```python
from build123d import *

# Parameters (mm, degrees)
F0_R     = 25.4
F1_DEPTH = 5.08
F3_DEPTH = 12.7
F4_R     = 1.5875
F5_DEPTH = 25.4


with BuildPart() as f1:
    # F0 (on Top) → F1 (new body)
    with BuildSketch(Plane.XY):
        Circle(F0_R)
    extrude(amount=F1_DEPTH)

    # F2 (on face) → F3 (join)
    with BuildSketch(Plane.XY.offset(5.08)):
        with BuildLine():
            ThreePointArc((13.335, 0), (0, -13.335), (-13.335, 0))
            Line((-13.335, 0), (-13.335, 12.7))
            ThreePointArc((-13.335, 12.7), (0, -18.415), (13.335, 12.7))
            Line((13.335, 12.7), (13.335, 0))
        make_face()
    extrude(amount=F3_DEPTH)

    # F4 (on face) → F5 (cut)
    with BuildSketch(Plane.XY.offset(5.08)):
        with Locations((-21.9075, 0)):
            Circle(F4_R)
        with Locations((21.9075, 0)):
            Circle(F4_R)
        with Locations((0, -21.9075)):
            Circle(F4_R)
    extrude(amount=-F5_DEPTH, mode=Mode.SUBTRACT)


solid = f1.part
```
Here's how the part is built. I have some questions about the finished solid (model axes, mm). A direction names the side the tool comes from. Round coordinates to 2 decimals unless told otherwise and drop trailing zeros. Loops run counter-clockwise (first coordinate to the right, second up) from the corner with the lowest first, then second, coordinate; pieces in that order, holes last. Notation, with made-up numbers: (44, 32) -> (69, 32) arc R21 ccw to (69, 52) -> close; hole circle Ø9 at (55.5, 27). An arc over 180 degrees is marked (long way). Answer as CSV lines item,"result". Start each with the question number.
1. Imagine slicing it at A-A on x = 0. Write out the boundary of the cut face in (y, z) (3 decimals), plus the area to 3 significant figures.
2. For faces 1 (the face through (13.335, 6, 11)), 2 (the face through (23.42, 0.48, 2.58)), 3 (the face through (-0.601, -18.405, 11.341)), which set-ups out of +Z, -Z, +X, -X, +Y, -Y let a thin tool reach every point of the face, with its end or its side?
3. Imagine slicing it at C-C on z = 11.5. Write out the boundary of the cut face in (x, y) (3 decimals), plus the area to 3 significant figures.
4. Imagine slicing it at B-B on y = 12. Write out the boundary of the cut face in (x, z) (3 decimals).
5. I need wall thicknesses on probe 1 along X at (y, z) = (-1, 2); probe 2 along Y at (x, z) = (0, 3.35) (3 decimals); probe 3 along Z at (x, y) = (5.5, 9.5). Which ranges of each line are inside material? Lowest first, please. Write a range as from..to.
6. I'm going to push flat-ended pins straight in: P1, Ø4, axis at y = 4, z = 7, coming from the -X side; P2, Ø2.5, axis at x = 0, y = -21.91, coming from the -Z side; P3, Ø8, axis at y = -9.5, z = 13, coming from the -X side; P4, Ø10, axis at x = -8.5, z = 3.5, coming from the +Y side. Where does each tip first touch, or does it pass through?
7. Imagine slicing it at D-D on x = -22. Write out the boundary of the cut face in (y, z), plus the area to 3 significant figures.
8. If we mould it in two halves opening along X, with no side actions, what happens to faces 4 (the face through (-2.8, -13.2, 17.78)), 5 (the face through (-23.493, 0.07, 2.576)), 6 (the face through (-5.506, -24.796, 2.504))? For each: pulls with the +X half, pulls with the -X half, needs draft (parallel to the pull), parting line crosses it, or undercut.
Solution:
1,outline,"(-25.4, 0) -> (-23.495, 0) -> (-23.495, 5.08) -> (-25.4, 5.08) -> close; (-20.32, 0) -> (25.4, 0) -> (25.4, 5.08) -> (-13.335, 5.08) -> (-13.335, 17.78) -> (-18.415, 17.78) -> (-18.415, 5.08) -> (-20.32, 5.08) -> close"
1,area,"306 mm²"
2,face 1,"+Z, +Y"
2,face 2,"+Z, -Z"
2,face 3,"+Z"
3,outline,"(-13.335, 0) -> (-13.335, 12.7) arc R18.415 ccw (long way) to (13.335, 12.7) -> (13.335, 0) arc R13.335 cw to start"
3,area,"342 mm²"
4,outline,"(-22.387, 0) -> (22.387, 0) -> (22.387, 5.08) -> (13.968, 5.08) -> (13.968, 17.78) -> (13.335, 17.78) -> (13.335, 5.08) -> (-13.335, 5.08) -> (-13.335, 17.78) -> (-13.968, 17.78) -> (-13.968, 5.08) -> (-22.387, 5.08) -> close"
5,probe 1,"-25.38..-23.14, -20.67..20.67, 23.14..25.38"
5,probe 2,"-25.4..-23.495, -20.32..25.4"
5,probe 3,"0..5.08"
6,P1,"x = -25.17"
6,P2,"through"
6,P3,"x = -17.57"
6,P4,"y = 25.16"
7,outline,"(-12.69, 0) -> (-1.58, 0) -> (-1.58, 5.08) -> (-12.69, 5.08) -> close; (1.58, 0) -> (12.69, 0) -> (12.69, 5.08) -> (1.58, 5.08) -> close"
7,area,"113 mm²"
8,face 4,"needs draft"
8,face 5,"undercut"
8,face 6,"parting line crosses it"
